Geometry check sheet. Reference: drawing and pictorial views, mm from the part's lowest x, y, z. Round coordinates to 2 decimals unless told otherwise and drop trailing zeros. Order: outer loops, then holes, each group sorted by start corner. A loop starts at its lowest first (then second) coordinate and runs counter-clockwise, first axis right, second up. Notation, with made-up numbers: (83.5, 21) -> (120.5, 21) arc R32 cw to (120.5, 47) -> close; hole circle Ø2 at (87.25, 77). An arc over 180 degrees is marked (long way). Return JSON: item names as keys, results as strings. Group by question number.
1) Section check C-C on y = 3.5. Enter the section's corners in (x, z), plus the area to 3 significant figures.
2) Draft check along Y on the marked faces 1, 2 and 3. Enter one of: pulls with the +Y half, pulls with the -Y half, needs draft (parallel to the pull), parting line crosses it, or undercut.
3) Section check D-D on x = 21.75. Enter the section's corners in (y, z), plus the area to 3 significant figures.
4) Section check B-B on z = 0.5. Enter the section's corners in (x, y).
5) Scan lines: L1, parallel to Y at x = 7.5, z = 2.5; L2, parallel to X at y = 3.5, z = 1.75; L3, parallel to X at y = 3.25, z = 2.25. Record each from-to range of solid material in increasing order.
6) Depth check by flat-ended pin: pin 1 (1.8 mm diameter, centred on x = 7.5, y = 3, fed in from -Z). Enter the tip coordinate at first touch or a pass-through.
7) Section check A-A on x = 15. Enter the section's corners in (y, z).
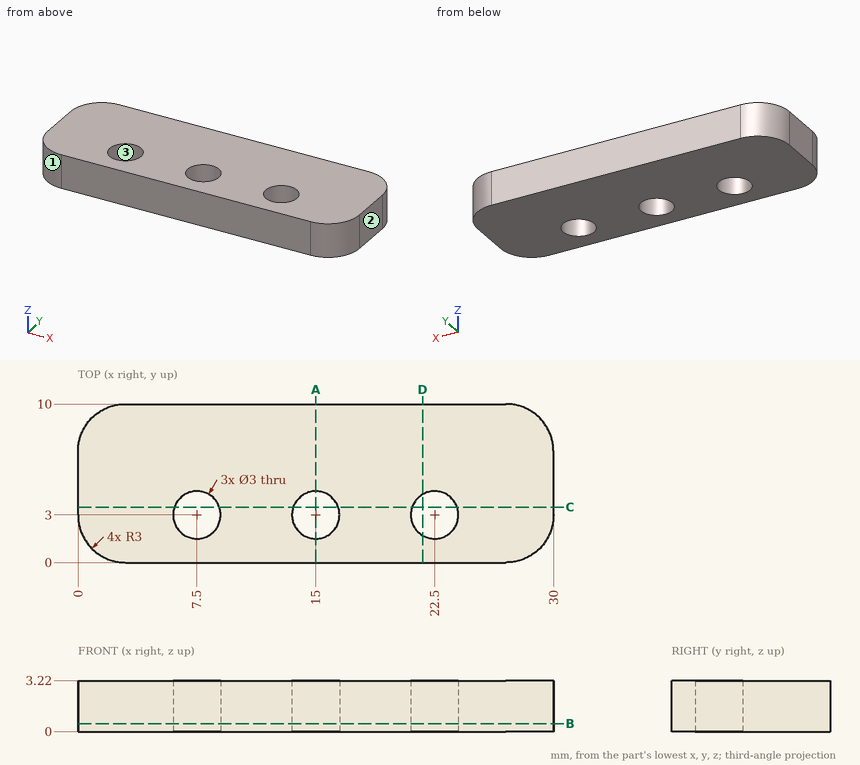
Check result:
{
 "1": {"outline": "(0, 0) -> (6.09, 0) -> (6.09, 3.22) -> (0, 3.22) -> close; (8.91, 0) -> (13.59, 0) -> (13.59, 3.22) -> (8.91, 3.22) -> close; (16.41, 0) -> (21.09, 0) -> (21.09, 3.22) -> (16.41, 3.22) -> close; (23.91, 0) -> (30, 0) -> (30, 3.22) -> (23.91, 3.22) -> close", "area": "69.3 mm^2"},
 "2": {"face 1": "pulls with the -Y half", "face 2": "needs draft", "face 3": "undercut"},
 "3": {"outline": "(0, 0) -> (1.7, 0) -> (1.7, 3.22) -> (0, 3.22) -> close; (4.3, 0) -> (10, 0) -> (10, 3.22) -> (4.3, 3.22) -> close", "area": "23.8 mm^2"},
 "4": {"outline": "(0, 3) arc R3 ccw to (3, 0) -> (27, 0) arc R3 ccw to (30, 3) -> (30, 7) arc R3 ccw to (27, 10) -> (3, 10) arc R3 ccw to (0, 7) -> close; hole circle Ø3 at (7.5, 3); hole circle Ø3 at (15, 3); hole circle Ø3 at (22.5, 3)"},
 "5": {"L1": "0 to 1.5, 4.5 to 10", "L2": "0 to 6.09, 8.91 to 13.59, 16.41 to 21.09, 23.91 to 30", "L3": "0 to 6.02, 8.98 to 13.52, 16.48 to 21.02, 23.98 to 30"},
 "6": {"pin 1": "through"},
 "7": {"outline": "(0, 0) -> (1.5, 0) -> (1.5, 3.22) -> (0, 3.22) -> close; (4.5, 0) -> (10, 0) -> (10, 3.22) -> (4.5, 3.22) -> close"}
}
